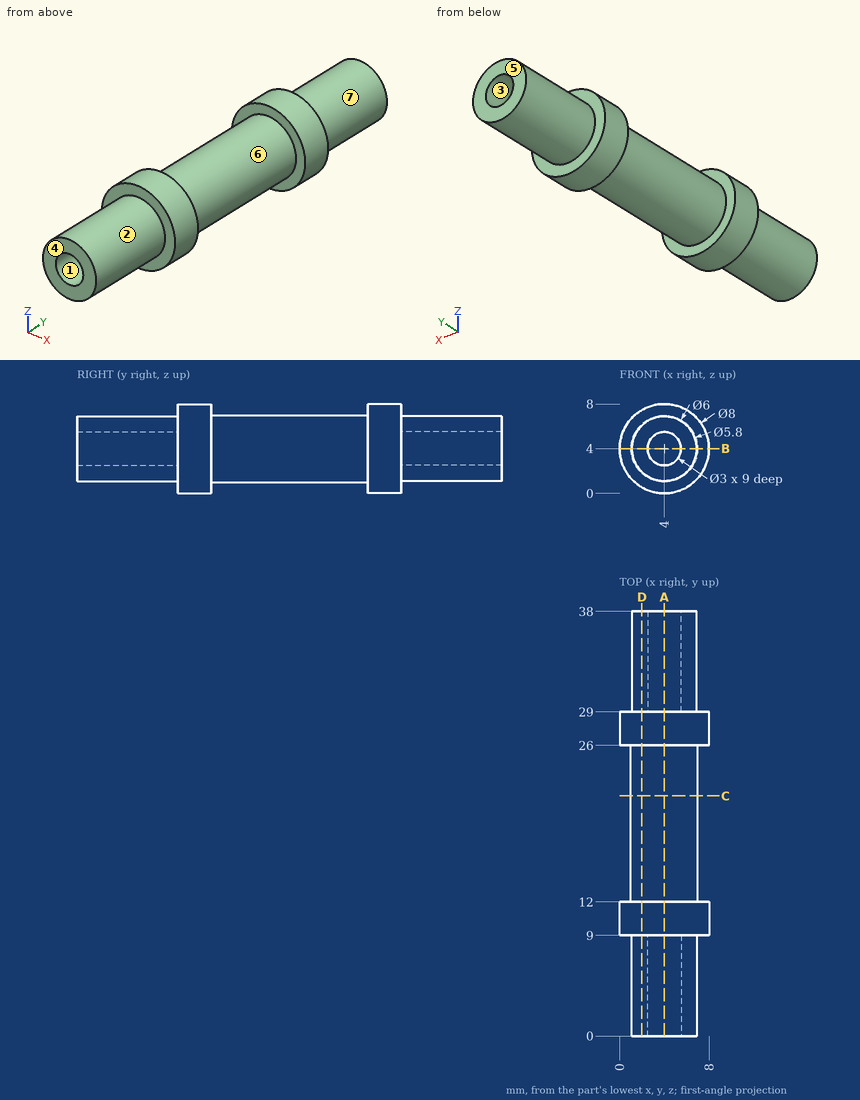
Geometry check sheet. Reference: drawing and pictorial views, mm from the part's lowest x, y, z. A direction names the side the tool comes from. Round coordinates to 2 decimals unless told otherwise and drop trailing zeros. Write each loop counter-clockwise with the first axis right and the second up, starting at its lowest first coordinate (ties: lowest second). Pieces come first, ordered by that corner, then holes. Notation, with made-up numbers: (5.25, -15.5) -> (41.25, -15.5) arc R22 cw to (41.25, -8.5) -> close; hole circle Ø1 at (16.5, -17). An arc over 180 degrees is marked (long way). One line per question, with ' | ' between items. Start each with the question number.
1. Sectioned sample at A-A, the plane x = 4. Record the cut outline in (y, z).
2. Sectioned sample at C-C, the plane y = 21.5. Record the cut outline in (x, z), then the cut area to 3 significant figures.
3. Release check for a two-part mould opening along X. For the marked faces 1, 2, 3 and 4 record: +X half, -X half, draft (parallel to the pull), parting line (faces both ways), or undercut.
4. Depth check by flat-ended pin: pin 1 (2.5 mm diameter, centred on x = 4, z = 4, fed in from +Y); pin 2 (0.9 mm diameter, centred on x = 4, z = 4.5, fed in from -Y); pin 3 (3 mm diameter, centred on y = 14.5, z = 7, fed in from +X). Enter the tip coordinate at first touch or a pass-through.
5. Set-up check for the marked faces 5, 6 and 7: record each of +Z, -Z, +X, -X, +Y, -Y from which the full face is reachable in a straight line by a thin tool's end or side.
6. Sectioned sample at B-B, the plane z = 4. Record the cut outline in (x, y), then the cut area to 3 significant figures.
7. Scan lines: line 1 along Z through (x, y) = (4, 32); line 2 along Y through (x, z) = (6, 6.5). Record each from-to range of solid material in increasing order. Write a range as from..to.
8. Sectioned sample at D-D, the plane x = 2. Record the cut outline in (y, z).
Taken from the geometry:
1) outline: (0, 1.1) -> (9, 1.1) -> (9, 0) -> (12, 0) -> (12, 1) -> (26, 1) -> (26, 0) -> (29, 0) -> (29, 1.1) -> (38, 1.1) -> (38, 2.5) -> (29, 2.5) -> (29, 5.5) -> (38, 5.5) -> (38, 6.9) -> (29, 6.9) -> (29, 8) -> (26, 8) -> (26, 7) -> (12, 7) -> (12, 8) -> (9, 8) -> (9, 6.9) -> (0, 6.9) -> (0, 5.5) -> (9, 5.5) -> (9, 2.5) -> (0, 2.5) -> close
2) outline: circle Ø6 at (4, 4) | area: 28.3 mm^2
3) face 1: undercut | face 2: parting line | face 3: undercut | face 4: draft
4) pin 1: stops at y = 29 | pin 2: stops at y = 9 | pin 3: stops at x = 6.6
5) face 5: +Z, -Z, +X, -X, +Y | face 6: none | face 7: +Y
6) outline: (0, 9) -> (1.1, 9) -> (1.1, 0) -> (2.5, 0) -> (2.5, 9) -> (5.5, 9) -> (5.5, 0) -> (6.9, 0) -> (6.9, 9) -> (8, 9) -> (8, 12) -> (7, 12) -> (7, 26) -> (8, 26) -> (8, 29) -> (6.9, 29) -> (6.9, 38) -> (5.5, 38) -> (5.5, 29) -> (2.5, 29) -> (2.5, 38) -> (1.1, 38) -> (1.1, 29) -> (0, 29) -> (0, 26) -> (1, 26) -> (1, 12) -> (0, 12) -> close | area: 182 mm^2
7) line 1: z = 1.1..2.5, 5.5..6.9 | line 2: y = 9..12, 26..29
8) outline: (0, 1.9) -> (9, 1.9) -> (9, 0.54) -> (12, 0.54) -> (12, 1.76) -> (26, 1.76) -> (26, 0.54) -> (29, 0.54) -> (29, 1.9) -> (38, 1.9) -> (38, 6.1) -> (29, 6.1) -> (29, 7.46) -> (26, 7.46) -> (26, 6.24) -> (12, 6.24) -> (12, 7.46) -> (9, 7.46) -> (9, 6.1) -> (0, 6.1) -> close
